Input: part model. Units: mm. Frame: model coordinates. A direction names the side the tool comes from. Coordinates: 2 decimals unless noted, no trailing zeros. Loops run counter-clockwise (first coordinate to the right, second up) from the corner with the lowest first, then second, coordinate; pieces in that order, holes last. Notation, with made-up numbers: (54, 45.25) -> (68, 45.25) arc R14 ccw to (68, 64.25) -> close; hole circle Ø10 at (61, 40.25). An arc over 180 degrees is marked (long way). Put each result on its own line as item: value. Start each with the question number.
1) Cut plane C-C (z = -6). Return the cut outline in (x, y) (3 decimals), plus the area to 3 significant figures.
2) Material intervals for L1, parallel to X at y = 3.05, z = -17; L2, parallel to X at y = 1.8, z = -16.5; L3, parallel to Y at x = -3, z = 9, sorted ascending.
3) Contact query for flat-ended pins moving along their axis: P1, Ø1, axis at x = 8.5, y = 4, coming from the +Z side; P2, Ø7, axis at x = 0, z = -6, coming from the +Y side; P3, Ø1.5, axis at y = 2.5, z = 2, coming from the -X side; P4, Ø2.5, axis at x = 0, z = 6, coming from the -Y side. Output: stop coordinate, or through.
4) Pull-direction query (X, two-part tool) for faces 6 (the flat face through (12.533, 2.535, 13.707)), 7 (the flat face through (-17.59, 2.54, 5.97)), 8 (the cylindrical face through (1.792, 1.014, -4.858)); classes: pulls with the +X half, pulls with the -X half, needs draft (parallel to the pull), parting line crosses it, or undercut.
5) Cut plane D-D (y = 1.5). State how many separate pieces and enclosed holes the cut face has, plus the area to 3 significant figures.
6) Cut plane B-B (x = -4.5). Return the cut outline in (y, z).
7) Cut plane A-A (z = -1). Return the cut outline in (x, y) (3 decimals), plus the area to 3 significant figures.
8) Set-up query: faces 1 (the flat face through (0, 0, 0)), 2 (the flat face through (14.446, 2.535, -11.764)), 3 (the flat face through (12.62, 2.54, -13.62)), 4 (the flat face through (-7.105, 2.535, 17.222)), 5 (the flat face through (-14.62, 2.54, -11.46)). Return all of +Z, -Z, +X, -X, +Y, -Y with unobstructed straight access to the full face (end or side cutting, diameter ignored); none if empty.
Autodesk Inventor part; units mm, degrees
ref_plane "YZ Plane" through (0, 0, 0) normal (1, 0, 0) x (0, 1, 0)
ref_plane "XZ Plane" through (0, 0, 0) normal (0, 1, 0) x (-1, 0, 0)
ref_plane "XY Plane" through (0, 0, 0) normal (0, 0, 1) x (1, 0, 0)
sketch "Sketch1" plane through (0, 0, 0) normal (0, 1, 0) x (-1, 0, 0)
  circle A0 centre (0, 0) radius 16.6257
  dimension "d0" = 33.2513
extrude "Extrusion1" add sketch "Sketch1" along normal blind 5
sketch "Sketch2" plane through (0, 5, 0) normal (0, 1, 0) x (1, 0, 0)
  circle A0 centre (0, 0) radius 10
  dimension "d3" = 20
extrude "Extrusion2" cut sketch "Sketch2" against normal blind 3
sketch "Sketch3" plane through (0, 2, 0) normal (0, 1, 0) x (1, 0, 0)
  circle A0 centre (-6, 0) radius 2.125
  circle A1 centre (-6, 0) radius 2.125
  point P0 (0, 0)
  dimension "d7" = 4.25
extrude "Extrusion3" cut sketch "Sketch3" against normal through all
pattern_circular "Circular Pattern1" count 4 over 360 about axis through (0, 5, 0) along (0, -1, 0) of "Extrusion3"
sketch "Sketch4" plane through (0, 2, 0) normal (0, 1, 0) x (1, 0, 0)
  circle A0 centre (0, 0) radius 2.125
  dimension "d13" = 4.25
extrude "Extrusion4" cut sketch "Sketch4" against normal blind 1
sketch "Sketch6" plane through (0, 5, 0) normal (0, 1, 0) x (1, 0, 0)
  arc A0 (5.4078, 16.6435) -> (0, 17.5) centre (0, 0) ccw
  line L0 (0, 0) -> (5.4078, 16.6435) construction
  line L1 (0, 0) -> (0, 17.5) construction
  line L2 (0, 0) -> (4.3015, 27.1585)
  line L3 (0, 0) -> (27.497, 0) construction
  arc A1 (5.4078, 16.6435) -> (0, 17.5) centre (0, 0) ccw
  dimension "d16" = 18
  dimension "d17" = 81
sketch "Sketch7" plane through (0, 5, 0) normal (0, 1, 0) x (1, 0, 0)
  circle A0 centre (0, 0) radius 16.6257
  arc A1 (5.1376, 15.8119) -> (0, 16.6257) centre (0, 0) ccw
  line L0 (0, 0) -> (5.1376, 15.8119) construction
  line L1 (0, 0) -> (0, 16.6257) construction
  line L2 (0, 0) -> (4.2807, 27.027)
  line L3 (0, 0) -> (27.3639, 0) construction
  line L4 (0, 16.6257) -> (3.2368, 20.4365)
  line L5 (3.2368, 20.4365) -> (5.1376, 15.8119)
  dimension "d18" = 18
  dimension "d19" = 81
  dimension "d20" = 5
extrude "Extrusion5" add sketch "Sketch7" against normal blind 5 contours A0 L2 L5 | L4 L2 A0
pattern_circular "Circular Pattern2" count 19 over 360 about axis through (0, 0, 0) along (0, 1, 0) of "Extrusion5"
sketch "Sketch8" plane through (0, 5, 0) normal (0, 1, 0) x (1, 0, 0)
  point P0 (0, 0)
sketch "Sketch9" plane through (0, 5, 0) normal (0, 1, 0) x (1, 0, 0)
  arc A0 (-12.044, -11.4609) -> (-7.9129, -14.6218) centre (0, 0) ccw
  line L0 (-7.9129, -14.6218) -> (-12.5734, -16.4328)
  line L1 (-7.9129, -14.6218) -> (-12.5734, -16.4328)
properties part number "SmallGearV2"
Results found:
1. outline: (-17.483, 0) -> (-2.125, 0) -> (-2.125, 2) -> (-8, 2) -> (-8, 5) -> (-17.483, 5) -> close; (2.125, 0) -> (17.183, 0) -> (17.183, 5) -> (8, 5) -> (8, 2) -> (2.125, 2) -> close
1. area: 117 mm2
2. L1: x = -10.05 to -8.05, -4.9 to -0.61, 0.32 to 4.65, 7.55 to 9.77
2. L2: x = -10.07 to -7.17, -5.09 to 4.85, 6.7 to 9.8
2. L3: y = 0 to 2
3. P1: stops at z = 14.8
3. P2: stops at y = 2
3. P3: stops at x = -17.61
3. P4: passes through
4. face 6: pulls with the +X half
4. face 7: pulls with the -X half
4. face 8: undercut
5. separate pieces: 1
5. enclosed holes: 5
5. area: 995 mm2
6. outline: (0, -18.02) -> (5, -18.02) -> (5, -8.93) -> (2, -8.93) -> (2, -1.51) -> (0, -1.51) -> close; (0, 1.51) -> (2, 1.51) -> (2, 8.93) -> (5, 8.93) -> (5, 17.89) -> (0, 17.89) -> close
7. outline: (-19.883, 0) -> (-7.875, 0) -> (-7.875, 2) -> (-9.95, 2) -> (-9.95, 5) -> (-19.883, 5) -> close; (-4.125, 0) -> (4.125, 0) -> (4.125, 2) -> (1.875, 2) -> (1.875, 1) -> (-1.875, 1) -> (-1.875, 2) -> (-4.125, 2) -> close; (7.875, 0) -> (19.42, 0) -> (19.42, 5) -> (9.95, 5) -> (9.95, 2) -> (7.875, 2) -> close
7. area: 118 mm2
8. face 1: +Z, -Z, +X, -X, -Y
8. face 2: +X, +Y, -Y
8. face 3: -Z, +Y, -Y
8. face 4: +Z, +Y, -Y
8. face 5: -X, +Y, -Y
